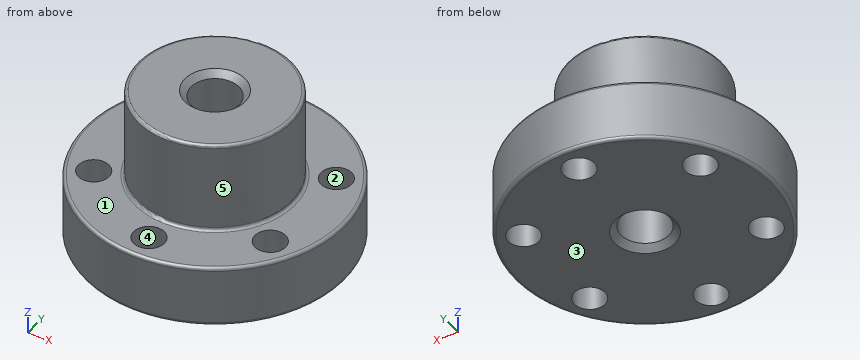
```python
from build123d import *

# Parameters (mm, degrees)
F2_R     = 2.5
F3_DEPTH = 25
F4_R     = 0.5
F5_SIZE  = 1


with BuildPart() as f1:
    # F0 (on Front) → F1 (revolve)
    with BuildSketch(Plane.XZ):
        Polygon((-21.055, 10), (-21.055, 0), (-3.9, 0), (-3.9, 24.8), (-12.5, 24.8), (-12.5, 10), align=None)
    revolve(axis=Axis((0, 0, 19.087244), (0, 0, 1)))

    # F2 (on face) → F3 (cut)
    with BuildSketch(Plane.XY.offset(10)):
        with Locations((0, 16.7775)):
            Circle(F2_R)
        with Locations((-14.529741, 8.38875)):
            Circle(F2_R)
        with Locations((-14.529741, -8.38875)):
            Circle(F2_R)
        with Locations((0, -16.7775)):
            Circle(F2_R)
        with Locations((14.529741, -8.38875)):
            Circle(F2_R)
        with Locations((14.529741, 8.38875)):
            Circle(F2_R)
    extrude(amount=-F3_DEPTH, mode=Mode.SUBTRACT)

    # F4
    f4_edges = [f1.edges().sort_by_distance(p)[0] for p in [
        (12.5, 0, 24.8),
        (21.055, 0, 10),
        (21.055, 0, 0),
        (12.5, 0, 10),
    ]]
    fillet(f4_edges, radius=F4_R)

    # F5
    f5_edges = [f1.edges().sort_by_distance(p)[0] for p in [
        (3.9, 0, 24.8),
        (3.9, 0, 0),
    ]]
    chamfer(f5_edges, length=F5_SIZE)


solid = f1.part
```
Input: part model. Units: mm. Frame: model coordinates. Face numbers are marked on the shaded views. A direction names the side the tool comes from. Coordinates: 2 decimals unless noted, no trailing zeros. Order: outer loops, then holes, each group sorted by start corner. A loop starts at its lowest first (then second) coordinate and runs counter-clockwise, first axis right, second up. Notation, with made-up numbers: (4, 47) - (25, 47) arc R12 ccw to (25, 61) - close; hole circle Ø8 at (23, 79.25). An arc over 180 degrees is marked (long way). Put each result on its own line as item: value.
1. Line query: line 1 along X through (y, z) = (0, 11); line 2 along X through (y, z) = (-8.5, 5.5); line 3 along Z through (x, y) = (-12, 15). Output: solid intervals per line, ascending.
Report:
line 1: x = -12.5 to -3.9, 3.9 to 12.5
line 2: x = -19.26 to -17.03, -12.03 to 12.03, 17.03 to 19.26
line 3: z = 0 to 10
2. Cut plane D-D on z = 13.75. Return the cut outline in (x, y).
Report:
outline: circle Ø25 at (0, 0); hole circle Ø7.8 at (0, 0)
3. Cut plane B-B on y = -9. State how many separate pieces and enclosed holes the cut face has, then the cut area to 3 significant figures.
Report:
separate pieces: 3
enclosed holes: 0
area: 540 mm2
4. Cut plane A-A on z = 4.75. Return the cut outline in (x, y) (1 decimal), then the cut area to 3 significant figures.
Report:
outline: circle Ø42.1 at (0, 0); hole circle Ø5 at (-14.5, -8.4); hole circle Ø5 at (-14.5, 8.4); hole circle Ø7.8 at (0, 0); hole circle Ø5 at (0, -16.8); hole circle Ø5 at (0, 16.8); hole circle Ø5 at (14.5, -8.4); hole circle Ø5 at (14.5, 8.4)
area: 1,230 mm2
5. Draft query along Y for the marked faces 3, 4 and 5. Return one class per face: pulls with the +Y half, pulls with the -Y half, needs draft (parallel to the pull), parting line crosses it, or undercut.
Report:
face 3: needs draft
face 4: undercut
face 5: parting line crosses it
6. Reachability of the marked faces 1 and 2 from +Z, -Z, +X, -X, +Y, -Y: full face, straight path, thin tool, end or side. Return the list, or none.
Report:
face 1: +Z
face 2: +Z, -Z
7. Contact query for flat-ended pins moving along their axis: pin 1 Ø6.5 at (x, y) = (-14.53, -8.39) entering from +Z; pin 2 Ø3 at (y, z) = (6, 13) entering from +X; pin 3 Ø3 at (x, z) = (1.5, 13.5) entering from +Y; pin 4 Ø4.5 at (x, y) = (-14.53, 8.39) entering from +Z. Output: stop coordinate, or through.
Report:
pin 1: stops at z = 10
pin 2: stops at x = 11.66
pin 3: stops at y = 12.5
pin 4: passes through
